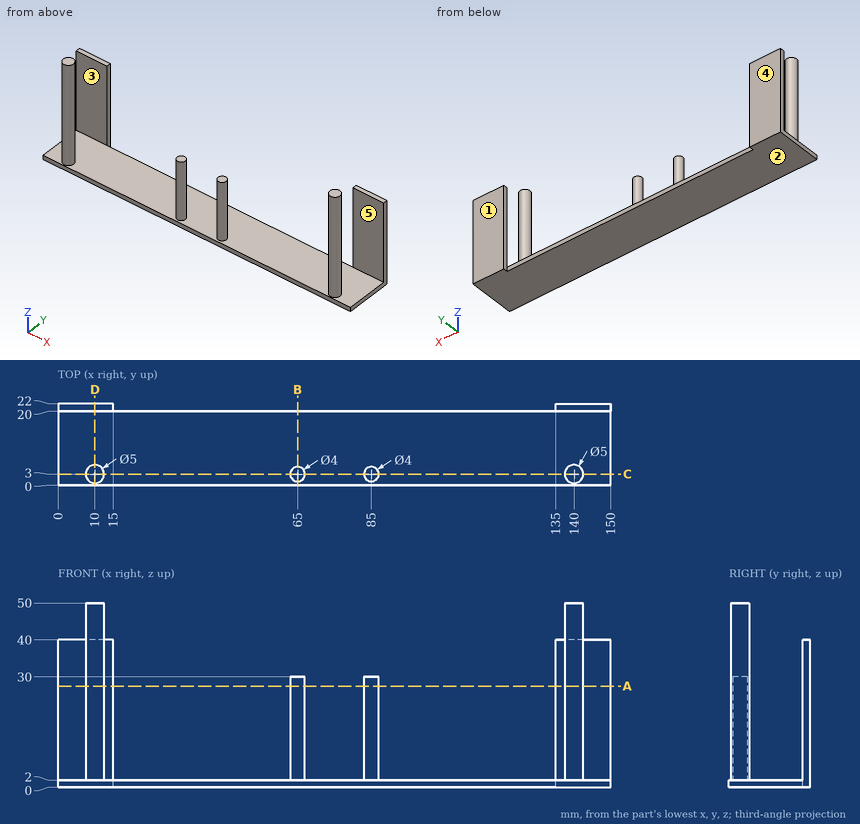
Source: three-view drawing plus pictorial views. Frame: mm from the lowest corner of the part. A direction names the side the tool comes from. Give positions to 0.01 mm unless a question says otherwise; leave off trailing zeros. Order: outer loops, then holes, each group sorted by start corner. A loop starts at its lowest first (then second) coordinate and runs counter-clockwise, first axis right, second up. Notation, with made-up numbers: M 25.5,72 L 76.5,72 A16 ccw 76.5,91 Z; hole C -27.5,37 d3. An arc over 180 degrees is marked long. One line per question, with ' | ' between items. Start each with the question number.
1. Pull-direction query (Y, two-part tool) for the marked faces 1, 2 and 3; classes: released by +Y, released by -Y, zero draft, split by the parting line, or undercut.
2. Section query C-C (y = 3). Return the cut outline in (x, z), and give its area (3 significant figures).
3. Section query B-B (x = 65). Return the cut outline in (y, z), and give its area (3 significant figures).
4. Material intervals for probe 1 along Z at (x, y) = (9, 18.25); probe 2 along Y at (x, z) = (7, 30.5); probe 3 along X at (y, z) = (3.75, 36.5), sorted ascending. Write a range as [from, to].
5. Section query A-A (z = 27.5). Return the cut outline in (x, y).
6. First-contact query: pin 1 Ø4 at (x, y) = (41.5, 4) entering from +Z; pin 2 Ø1.6 at (x, z) = (102, 1) entering from +Y; pin 3 Ø1 at (x, y) = (11, 21.5) entering from +Z. Flat tips, straight axial feed; report the tip coordinate or a pass-through.
7. Section query D-D (x = 10). Return the cut outline in (y, z), and give its area (3 significant figures).
8. Access query for the marked faces 4 and 5. Directions: +Z, -Z, +X, -X, +Y, -Y. A direction counts if a zero-diameter tool reaches every point of the face in a straight line with its end or side. Return the directions, or none.
Here are the results:
1) face 1: released by +Y | face 2: zero draft | face 3: undercut
2) outline: M 0,0 L 150,0 L 150,2 L 142.5,2 L 142.5,50 L 137.5,50 L 137.5,2 L 87,2 L 87,30 L 83,30 L 83,2 L 67,2 L 67,30 L 63,30 L 63,2 L 12.5,2 L 12.5,50 L 7.5,50 L 7.5,2 L 0,2 Z | area: 1,000 mm²
3) outline: M 0,0 L 20,0 L 20,2 L 5,2 L 5,30 L 1,30 L 1,2 L 0,2 Z | area: 152 mm²
4) probe 1: [0, 2] | probe 2: [20, 22] | probe 3: [7.62, 12.38], [137.62, 142.38]
5) outline: M 0,20 L 15,20 L 15,22 L 0,22 Z; C 10,3 d5; C 65,3 d4; C 85,3 d4; M 135,20 L 150,20 L 150,22 L 135,22 Z; C 140,3 d5
6) pin 1: z = 2 | pin 2: y = 20 | pin 3: z = 40
7) outline: M 0,0 L 22,0 L 22,40 L 20,40 L 20,2 L 5.5,2 L 5.5,50 L 0.5,50 L 0.5,2 L 0,2 Z | area: 360 mm²
8) face 4: +Z, -Z, +X, -X, +Y | face 5: +Z, +X, -X
